```python
from build123d import *

# Parameters (mm, degrees)
SKETCH1_W                 = 304.8
SKETCH1_H                 = 25.4
BOSS_EXTRUDE2_DEPTH       = 12.7
FILLET1_R                 = 12.7
CUT_EXTRUDE3_DEPTH        = 281.209703849
SKETCH8_W                 = 70
SKETCH8_H                 = 25.4
BOSS_EXTRUDE3_DEPTH       = 9.7
CUT_EXTRUDE4_DEPTH        = 281.209703849
CUT_EXTRUDE5_DEPTH        = 281.209703849
SKETCH13_W                = 12.7
SKETCH13_H                = 25.4
CUT_EXTRUDE7_DEPTH        = 280.450243045
F_6_CLEARANCE_HOLE1_D     = 3.7973
F_6_CLEARANCE_HOLE1_DEPTH = 3


with BuildPart() as part:
    # Sketch1 → Boss-Extrude2 (new body)
    with BuildSketch(Plane.XY):
        with Locations((126.366978193, -2.136448598)):
            Rectangle(SKETCH1_W, SKETCH1_H)
    extrude(amount=BOSS_EXTRUDE2_DEPTH)

    # Fillet1
    fillet1_edges = [part.edges().sort_by_distance(p)[0] for p in [
        (-26.033021807, -2.136448598, 12.7),
        (278.766978193, -2.136448598, 12.7),
    ]]
    fillet(fillet1_edges, radius=FILLET1_R - 0.0001)  # a hair under: the kernel refuses the full size

    # Sketch6 → Cut-Extrude3 (cut, through all)
    with BuildSketch(Plane(origin=(0, 10.563551402, 0), x_dir=(1, 0, 0), z_dir=(0, 1, 0))):
        with BuildLine():
            Line((-23.033021807, 0), (275.766978193, 0))
            ThreePointArc((275.766978193, 0), (272.925913971, -6.858935778), (266.066978193, -9.7))
            Line((266.066978193, -9.7), (-13.333021807, -9.7))
            ThreePointArc((-13.333021807, -9.7), (-20.191957584, -6.858935778), (-23.033021807, 0))
        make_face()
    extrude(amount=-CUT_EXTRUDE3_DEPTH, mode=Mode.SUBTRACT)

    # Sketch8 → Boss-Extrude3 (add)
    with BuildSketch(Plane(origin=(0, 0, 9.7), x_dir=(-1, 0, 0), z_dir=(0, 0, -1))):
        with Locations((-180.266978193, -2.136448598)):
            Rectangle(SKETCH8_W, SKETCH8_H)
        with Locations((-72.466978193, -2.136448598)):
            Rectangle(SKETCH8_W, SKETCH8_H)
    extrude(amount=BOSS_EXTRUDE3_DEPTH)

    # Sketch9 → Cut-Extrude4 (cut, through all)
    with BuildSketch(Plane(origin=(0, 10.563551402, 0), x_dir=(1, 0, 0), z_dir=(0, 1, 0))):
        Polygon((145.266978193, -9.7), (165.266978193, -9.7), (192.266978193, -9.7), (165.266978193, -3), (145.266978193, -3), align=None)
        Polygon((215.266978193, -6.7), (195.266978193, -6.7), (168.266978193, 0), (215.266978193, 0), align=None)
    extrude(amount=-CUT_EXTRUDE4_DEPTH, mode=Mode.SUBTRACT)

    # Sketch12 → Cut-Extrude5 (cut, through all)
    with BuildSketch(Plane(origin=(0, 10.563551402, 0), x_dir=(1, 0, 0), z_dir=(0, 1, 0))):
        Polygon((107.466978193, -9.7), (107.466978193, -3), (87.466978193, -3), (60.466978193, -9.7), align=None)
        Polygon((37.466978193, -6.7), (57.466978193, -6.7), (84.466978193, 0), (37.466978193, 0), align=None)
    extrude(amount=-CUT_EXTRUDE5_DEPTH, mode=Mode.SUBTRACT)

    # Sketch13 → Cut-Extrude7 (cut, through all)
    with BuildSketch(Plane.XY.offset(12.7)):
        with Locations((-19.683021807, -2.136448598)):
            Rectangle(SKETCH13_W, SKETCH13_H)
        with Locations((272.416978193, -2.136448598)):
            Rectangle(SKETCH13_W, SKETCH13_H)
    extrude(amount=-CUT_EXTRUDE7_DEPTH, mode=Mode.SUBTRACT)

    # #6 Clearance Hole1
    with Locations(Plane.XY.offset(3)):
        with Locations((97.466978193, 5.363551402), (97.466978193, -9.636448598), (155.266978193, -9.636448598), (155.266978193, 5.363551402)):
            Hole(F_6_CLEARANCE_HOLE1_D / 2, depth=F_6_CLEARANCE_HOLE1_DEPTH)


solid = part.part
```
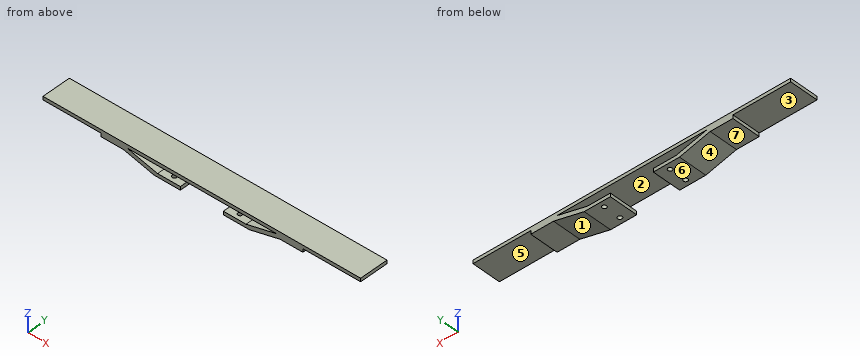
Input: part model. Units: mm. Frame: model coordinates. Face numbers are marked on the shaded views. A direction names the side the tool comes from. Coordinates: 2 decimals unless noted, no trailing zeros. Write each loop counter-clockwise with the first axis right and the second up, starting at its lowest first coordinate (ties: lowest second). Pieces come first, ordered by that corner, then holes.
1) Set-up query: the marked faces 5, 6 and 7. Return all of +Z, -Z, +X, -X, +Y, -Y with unobstructed straight access to the full face (end or side cutting, diameter ignored); none if empty.
2) Section B-B on y = -1.25. Output: boundary loops of the cut face in (x, z).
3) Section A-A on x = 182. Output: boundary loops of the cut face in (y, z), and give its area (3 significant figures).
4) Material intervals for line 1 along Z through (x, y) = (163, 4.5); line 2 along Z through (x, y) = (28, 6); line 3 along Z through (x, y) = (182, 0), sorted ascending.
5) Mould query, pull axis X, two halves, no side actions, for the marked faces 1, 2, 3 and 4. Classes: pulls with the +X half, pulls with the -X half, needs draft (parallel to the pull), parting line crosses it, or undercut.
6) Pin query (flat end, axial travel): pin 1 Ø10 at (x, y) = (208, 2) entering from -Z; pin 2 Ø5 at (x, y) = (97.47, 5.36) entering from -Z; pin 3 Ø12.5 at (x, y) = (120.5, -3.5) entering from -Z; pin 4 Ø5 at (y, z) = (-8.5, 5) entering from +X. Return the tip coordinate at first contact, or that it passes through.
7) Section C-C on x = 31. Output: boundary loops of the cut face in (y, z).
Check result:
1. face 5: -Z, +X, +Y, -Y
1. face 6: -Z, +X, -X, +Y, -Y
1. face 7: -Z, -X, +Y, -Y
2. outline: (-13.33, 9.7) - (37.47, 9.7) - (37.47, 6.7) - (57.47, 6.7) - (84.47, 0) - (107.47, 0) - (107.47, 3) - (87.47, 3) - (60.47, 9.7) - (192.27, 9.7) - (165.27, 3) - (145.27, 3) - (145.27, 0) - (168.27, 0) - (195.27, 6.7) - (215.27, 6.7) - (215.27, 9.7) - (266.07, 9.7) - (266.07, 12.7) - (-13.33, 12.7) - close
3. outline: (-14.84, 3.41) - (10.56, 3.41) - (10.56, 7.15) - (-14.84, 7.15) - close; (-14.84, 9.7) - (10.56, 9.7) - (10.56, 12.7) - (-14.84, 12.7) - close
3. area: 171 mm2
4. line 1: z = 0 to 3, 9.7 to 12.7
4. line 2: z = 9.7 to 12.7
4. line 3: z = 3.41 to 7.15, 9.7 to 12.7
5. face 1: pulls with the +X half
5. face 2: undercut
5. face 3: needs draft
5. face 4: pulls with the -X half
6. pin 1: stops at z = 6.7
6. pin 2: stops at z = 0
6. pin 3: stops at z = 9.7
6. pin 4: stops at x = 215.27
7. outline: (-14.84, 9.7) - (10.56, 9.7) - (10.56, 12.7) - (-14.84, 12.7) - close
